Input: part model. Units: mm. Frame: model coordinates. A direction names the side the tool comes from. Give positions to 0.01 mm unless a question says otherwise; leave off trailing zeros. Loops run counter-clockwise (first coordinate to the right, second up) from the corner with the lowest first, then second, coordinate; pieces in that order, holes last. Notation, with made-up numbers: M 55.25,59 L 111.25,59 A16 ccw 111.25,64 Z; hole C -35.5,4.25 d11. An arc over 180 degrees is marked long. Answer as a JSON object with one key per item and string values. Group by question number.
1) Section query B-B on y = -19. Return loops of the section in (x, z) (3 decimals), plus the area to 3 significant figures.
2) Ray query, L1, parallel to Z at x = 6, y = -18.5 (3 decimals); L2, parallel to Y at x = 3.5, z = 8. Return the intervals inside material, ascending.
3) Section query A-A on x = -2. Return loops of the section in (y, z) (3 decimals), plus the area to 3 significant figures.
4) Access query for faces 4 (the flat face through (8, -24.108, 13)), 5 (the flat face through (8, -20.933, 14)). Directions: +Z, -Z, +X, -X, +Y, -Y. A direction counts if a zero-diameter tool reaches every point of the face in a straight line with its end or side. Return the directions, or none.
5) First-contact query: P1, Ø9, axis at x = 7.5, z = 16.5, coming from the +Y side; P2, Ø1.8, axis at x = 20.03, z = 26.18, coming from the +Y side; P3, Ø8, axis at x = 10.5, y = -7.5, coming from the +Z side. Flat tips, straight axial feed; report the tip coordinate or a pass-through.
6) Draft query along Z for faces 1 (the flat face through (8, -5, 0)), 2 (the cylindrical face through (18.7, -22.5, 26.87)), 3 (the flat face through (8, 11.452, -2)). Return one class per face: +Z half, -Z half, draft (parallel to the pull), parting line (faces both ways), or undercut.
7) Section query C-C on z = 22. Return loops of the section in (x, y).
8) Section query D-D on x = 25.5. Return loops of the section in (y, z) (3 decimals).
from build123d import *

# Parameters (mm, degrees)
SKETCH1_W                  = 38.1
SKETCH1_H                  = 10.16
SKETCH1_R                  = 1.27
BOSS_EXTRUDE3_DEPTH        = 3.175
SKETCH7_W                  = 38.1
SKETCH7_H                  = 3.175
BOSS_EXTRUDE4_DEPTH        = 25.4
SKETCH8_W                  = 38.1
SKETCH8_H                  = 3.175
BOSS_EXTRUDE6_DEPTH        = 29.21
F_1_0_228_DIAMETER_HOLE1_D = 3.000000096


with BuildPart() as part:
    # Sketch1 → Boss-Extrude3 (new body)
    with BuildSketch(Plane.XY):
        with Locations((8.461414392, 6.372059553)):
            Rectangle(SKETCH1_W, SKETCH1_H)
        with Locations((16.081414392, 6.372059553)):
            Circle(SKETCH1_R, mode=Mode.SUBTRACT)
        with Locations((0.841414392, 6.372059553)):
            Circle(SKETCH1_R, mode=Mode.SUBTRACT)
    extrude(amount=-BOSS_EXTRUDE3_DEPTH)

    # Sketch7 → Boss-Extrude4 (add)
    with BuildSketch(Plane.XZ.offset(-1.292059553)):
        with Locations((8.461414392, -1.5875)):
            Rectangle(SKETCH7_W, SKETCH7_H)
    extrude(amount=BOSS_EXTRUDE4_DEPTH)

    # Sketch8 → Boss-Extrude6 (add)
    with BuildSketch(Plane.XY):
        with Locations((8.461414392, -22.520440447)):
            Rectangle(SKETCH8_W, SKETCH8_H)
    extrude(amount=BOSS_EXTRUDE6_DEPTH)

    # #1 (0.228) Diameter Hole1 (through all)
    with Locations(Plane(origin=(-2.968585608, -24.107940447, 3.175), x_dir=(0, 0, -1), z_dir=(0, -1, 0))):
        with Locations((0, 0), (0, 23), (-23, 23), (-23, 0)):
            Hole(F_1_0_228_DIAMETER_HOLE1_D / 2)


solid = part.part
Output:
{
 "1": {"outline": "M -10.589,-3.175 L 27.511,-3.175 L 27.511,0 L -10.589,0 Z", "area": "121 mm^2"},
 "2": {"L1": "z = -3.175 to 0", "L2": "y = -24.11 to -20.93"},
 "3": {"outline": "M -24.108,-3.175 L 11.452,-3.175 L 11.452,0 L -20.933,0 L -20.933,2.03 L -24.108,2.03 Z; M -24.108,4.32 L -20.933,4.32 L -20.933,25.03 L -24.108,25.03 Z; M -24.108,27.32 L -20.933,27.32 L -20.933,29.21 L -24.108,29.21 Z", "area": "191 mm^2"},
 "4": {"face 4": "+Z, -Z, +X, -X, -Y", "face 5": "+Z, +X, -X, +Y"},
 "5": {"P1": "stops at y = -20.93", "P2": "passes through", "P3": "stops at z = 0"},
 "6": {"face 1": "+Z half", "face 2": "undercut", "face 3": "draft"},
 "7": {"outline": "M -10.59,-24.11 L 27.51,-24.11 L 27.51,-20.93 L -10.59,-20.93 Z"},
 "8": {"outline": "M -24.108,-3.175 L 11.452,-3.175 L 11.452,0 L -20.933,0 L -20.933,29.21 L -24.108,29.21 Z"}
}
